from build123d import *

# Parameters (mm, degrees)
SALIENTE_EXTRUIR1_DEPTH      = 50
SALIENTE_EXTRUIR1_DEPTH_BACK = 7
CROQUIS1_W                   = 20
CROQUIS1_H                   = 20
CROQUIS2_R                   = 4
CORTAR_EXTRUIR1_DEPTH        = 58.445626465
CORTAR_EXTRUIR2_DEPTH        = 5
CROQUIS4_R                   = 4
CORTAR_EXTRUIR3_DEPTH        = 58.445626465
CORTAR_EXTRUIR4_DEPTH        = 5
REDONDEO1_R                  = 5
REDONDEO2_R                  = 1
REDONDEO3_R                  = 1


with BuildPart() as part:
    # Croquis1 → Saliente-Extruir1 (new, two sides: drawn at the far end of the back side and taken through both)
    with BuildSketch(Plane(origin=(0, 0, 0), x_dir=(1, 0, 0), z_dir=(0, 1, 0)).offset(-SALIENTE_EXTRUIR1_DEPTH_BACK)):
        with Locations((10, 10)):
            Rectangle(CROQUIS1_W, CROQUIS1_H)
    extrude(amount=SALIENTE_EXTRUIR1_DEPTH + SALIENTE_EXTRUIR1_DEPTH_BACK)

    # Croquis2 → Cortar-Extruir1 (cut, through all)
    with BuildSketch(Plane.XY):
        with Locations((10, 45)):
            Circle(CROQUIS2_R)
        with Locations((10, 20)):
            Circle(CROQUIS2_R)
    extrude(amount=-CORTAR_EXTRUIR1_DEPTH, mode=Mode.SUBTRACT)

    # Croquis3 → Cortar-Extruir2 (cut)
    with BuildSketch(Plane.XY):
        Polygon((13.92598183, 26.8), (6.07401817, 26.8), (2.148036339, 20), (6.07401817, 13.2), (13.92598183, 13.2), (17.851963661, 20), align=None)
    extrude(amount=-CORTAR_EXTRUIR2_DEPTH, mode=Mode.SUBTRACT)

    # Croquis4 → Cortar-Extruir3 (cut, through all)
    with BuildSketch(Plane.ZY):
        with Locations((-10, 30)):
            Circle(CROQUIS4_R)
        with Locations((-10, 10)):
            Circle(CROQUIS4_R)
    extrude(amount=-CORTAR_EXTRUIR3_DEPTH, mode=Mode.SUBTRACT)

    # Croquis5 → Cortar-Extruir4 (cut)
    with BuildSketch(Plane.ZY):
        Polygon((-6.07401817, 23.2), (-2.148036339, 30), (-6.07401817, 36.8), (-13.92598183, 36.8), (-17.851963661, 30), (-13.92598183, 23.2), align=None)
        Polygon((-6.07401817, 16.8), (-13.92598183, 16.8), (-17.851963661, 10), (-13.92598183, 3.2), (-6.07401817, 3.2), (-2.148036339, 10), align=None)
    extrude(amount=-CORTAR_EXTRUIR4_DEPTH, mode=Mode.SUBTRACT)

    # Redondeo1
    redondeo1_edges = [part.edges().sort_by_distance(p)[0] for p in [
        (0, 50, -10),
        (20, 50, -10),
    ]]
    fillet(redondeo1_edges, radius=REDONDEO1_R)

    # Redondeo2
    redondeo2_edges = [part.edges().sort_by_distance(p)[0] for p in [
        (20, -7, -10),
        (10, -7, -20),
        (0, -7, -10),
        (10, -7, 0),
    ]]
    fillet(redondeo2_edges, radius=REDONDEO2_R)

    # Redondeo3
    # the kernel refuses this fillet: 1 mm, written as the material it takes off along each edge
    with BuildSketch(Plane(origin=(19, -6, -19), x_dir=(0, 0, -1), z_dir=(1, 0, 0))) as redondeo3_piece_1_section:
        Polygon((0, 0), (REDONDEO3_R, 0), (REDONDEO3_R, -REDONDEO3_R), (0, -REDONDEO3_R), align=None)
    redondeo3_piece_1 = extrude(amount=REDONDEO3_R, mode=Mode.PRIVATE)
    redondeo3_piece_1 = redondeo3_piece_1 - Plane(origin=(19, -6, -19), x_dir=(0, 0.7071067811865475, 0.7071067811865475), z_dir=(1, 0, 0)) * Sphere(REDONDEO3_R, mode=Mode.PRIVATE)
    add(redondeo3_piece_1, mode=Mode.SUBTRACT)
    with BuildSketch(Plane(origin=(19, -6, -1), x_dir=(1, 0, 0), z_dir=(0, 0, 1))) as redondeo3_piece_2_section:
        Polygon((0, 0), (REDONDEO3_R, 0), (REDONDEO3_R, -REDONDEO3_R), (0, -REDONDEO3_R), align=None)
    redondeo3_piece_2 = extrude(amount=REDONDEO3_R, mode=Mode.PRIVATE)
    redondeo3_piece_2 = redondeo3_piece_2 - Plane(origin=(19, -6, -1), x_dir=(-0.7071067811865475, 0.7071067811865475, 0), z_dir=(0, 0, 1)) * Sphere(REDONDEO3_R, mode=Mode.PRIVATE)
    add(redondeo3_piece_2, mode=Mode.SUBTRACT)
    with BuildSketch(Plane(origin=(1, -6, -19), x_dir=(0, 0, -1), z_dir=(-1, 0, 0))) as redondeo3_piece_3_section:
        Polygon((0, 0), (REDONDEO3_R, 0), (REDONDEO3_R, REDONDEO3_R), (0, REDONDEO3_R), align=None)
    redondeo3_piece_3 = extrude(amount=REDONDEO3_R, mode=Mode.PRIVATE)
    redondeo3_piece_3 = redondeo3_piece_3 - Plane(origin=(1, -6, -19), x_dir=(0, 0.7071067811865475, 0.7071067811865475), z_dir=(-1, 0, 0)) * Sphere(REDONDEO3_R, mode=Mode.PRIVATE)
    add(redondeo3_piece_3, mode=Mode.SUBTRACT)
    with BuildSketch(Plane(origin=(1, -6, -1), x_dir=(-1, 0, 0), z_dir=(0, 0, 1))) as redondeo3_piece_4_section:
        Polygon((0, 0), (REDONDEO3_R, 0), (REDONDEO3_R, REDONDEO3_R), (0, REDONDEO3_R), align=None)
    redondeo3_piece_4 = extrude(amount=REDONDEO3_R, mode=Mode.PRIVATE)
    redondeo3_piece_4 = redondeo3_piece_4 - Plane(origin=(1, -6, -1), x_dir=(0.7071067811865475, 0.7071067811865475, 0), z_dir=(0, 0, 1)) * Sphere(REDONDEO3_R, mode=Mode.PRIVATE)
    add(redondeo3_piece_4, mode=Mode.SUBTRACT)
    with BuildSketch(Plane(origin=(5, 50, 0), x_dir=(0, -1, 0), z_dir=(1, 0, 0))) as redondeo3_piece_5:
        with BuildLine():
            CenterArc((REDONDEO3_R, REDONDEO3_R), REDONDEO3_R, 180, 90)
            Line((0, REDONDEO3_R), (0, 0))
            Line((0, 0), (REDONDEO3_R, 0))
        make_face()
    extrude(amount=10, mode=Mode.SUBTRACT)
    with BuildSketch(Plane(origin=(15, 50, -20), x_dir=(0, 0, 1), z_dir=(-1, 0, 0))) as redondeo3_piece_6:
        with BuildLine():
            CenterArc((REDONDEO3_R, -REDONDEO3_R), REDONDEO3_R, 90, 90)
            Line((0, -REDONDEO3_R), (0, 0))
            Line((0, 0), (REDONDEO3_R, 0))
        make_face()
    extrude(amount=10, mode=Mode.SUBTRACT)
    with BuildSketch(Plane(origin=(5, 45, -20), x_dir=(-1, 0, 0), z_dir=(0, -1, 0))) as redondeo3_piece_7:
        with BuildLine():
            CenterArc((5 - REDONDEO3_R, -REDONDEO3_R), REDONDEO3_R, 0, 90)
            Line((5 - REDONDEO3_R, 0), (5, 0))
            Line((5, 0), (5, -REDONDEO3_R))
        make_face()
    revolve(axis=Axis((5, 45, -20), (0, 0, -1)), revolution_arc=90, mode=Mode.SUBTRACT)
    with BuildSketch(Plane(origin=(15, 45, -20), x_dir=(0, 1, 0), z_dir=(-1, 0, 0))) as redondeo3_piece_8:
        with BuildLine():
            CenterArc((5 - REDONDEO3_R, -REDONDEO3_R), REDONDEO3_R, 0, 90)
            Line((5 - REDONDEO3_R, 0), (5, 0))
            Line((5, 0), (5, -REDONDEO3_R))
        make_face()
    revolve(axis=Axis((15, 45, -20), (0, 0, -1)), revolution_arc=90, mode=Mode.SUBTRACT)
    with BuildSketch(Plane(origin=(5, 45, 0), x_dir=(-1, 0, 0), z_dir=(0, -1, 0))) as redondeo3_piece_9:
        with BuildLine():
            CenterArc((5 - REDONDEO3_R, REDONDEO3_R), REDONDEO3_R, 270, 90)
            Line((5, REDONDEO3_R), (5, 0))
            Line((5, 0), (5 - REDONDEO3_R, 0))
        make_face()
    revolve(axis=Axis((5, 45, 0), (0, 0, -1)), revolution_arc=90, mode=Mode.SUBTRACT)
    with BuildSketch(Plane(origin=(15, 45, 0), x_dir=(0, 1, 0), z_dir=(-1, 0, 0))) as redondeo3_piece_10:
        with BuildLine():
            CenterArc((5 - REDONDEO3_R, REDONDEO3_R), REDONDEO3_R, 270, 90)
            Line((5, REDONDEO3_R), (5, 0))
            Line((5, 0), (5 - REDONDEO3_R, 0))
        make_face()
    revolve(axis=Axis((15, 45, 0), (0, 0, -1)), revolution_arc=90, mode=Mode.SUBTRACT)
    with BuildSketch(Plane(origin=(0, 45, 0), x_dir=(1, 0, 0), z_dir=(0, -1, 0)), Plane(origin=(0, 45, -20), x_dir=(0, 0, 1), z_dir=(0, -1, 0)), Plane(origin=(20, -6, -20), x_dir=(0, 0, 1), z_dir=(0, 1, 0)), Plane(origin=(20, -6, 0), x_dir=(-1, 0, 0), z_dir=(0, 1, 0))) as redondeo3_piece_11:
        with BuildLine():
            CenterArc((REDONDEO3_R, -REDONDEO3_R), REDONDEO3_R, 90, 90)
            Line((0, -REDONDEO3_R), (0, 0))
            Line((0, 0), (REDONDEO3_R, 0))
        make_face()
    extrude(amount=51, mode=Mode.SUBTRACT)


solid = part.part
Source: CAD feature listing. Evaluate the final solid. Frame: model axes, mm. A direction names the side the tool comes from. Round coordinates to 2 decimals unless told otherwise and drop trailing zeros. Loops run counter-clockwise (first coordinate to the right, second up) from the corner with the lowest first, then second, coordinate; pieces in that order, holes last. Notation, with made-up numbers: (23.5, 89.25) -> (75.5, 89.25) arc R3 cw to (75.5, 94.25) -> close; hole circle Ø10 at (-30.5, 70.25). An arc over 180 degrees is marked (long way). Answer as a JSON object with one key per item and string values. Group by question number.
Q1. Section query D-D (x = 17). State how many separate pieces and enclosed holes the cut face has, plus the area to 3 significant figures.
Q2. Contact query for flat-ended pins moving along their axis: P1, Ø1.5, axis at x = 2, z = -10.5, coming from the +Y side; P2, Ø4, axis at x = 7, y = 17, coming from the +Z side; P3, Ø10, axis at y = 11, z = -11, coming from the -X side. Output: stop coordinate, or through.
Q3. Section query B-B (z = -11.5). Output: boundary loops of the cut face in (x, y).
Q4. Section query A-A (x = 8.25). Output: boundary loops of the cut face in (y, z).
Q5. Ray query, line 1 (Y direction, x = 14.5, z = -9.25); line 2 (Y direction, x = 11, z = -12.75); line 3 (Y direction, x = 14.75, z = -12.5). Return the intervals inside material, ascending. Write a range as from..to.
Q6. Access query for faces 4 (the flat face through (15.92, 23.35, -2.46)), 5 (the cylindrical face through (0.285, 19.857, -19.699)), 6 (the flat face through (2.46, 33.35, -4.08)). Directions: +Z, -Z, +X, -X, +Y, -Y. A direction counts if a zero-diameter tool reaches every point of the face in a straight line with its end or side. Return the directions, or none.
Q7. Mould query, pull axis Z, two halves, no side actions, for faces 1 (the flat face through (2, 23.2, -10)), 2 (the flat face through (15.86, 16.55, -2.46)), 3 (the flat face through (5.9, 21.1, -20)). Classes: pulls with the +Z half, pulls with the -Z half, needs draft (parallel to the pull), parting line crosses it, or undercut.
Q8. Section query C-C (y = 8.5). Output: boundary loops of the cut face in (x, z), plus the area to 3 significant figures.
Completed:
{
 "1": {"separate pieces": "1", "enclosed holes": "2", "area": "1,020 mm²"},
 "2": {"P1": "y = 49.47", "P2": "z = -5", "P3": "x = 5"},
 "3": {"outline": "(0, -6) arc R1 ccw to (1, -7) -> (19, -7) arc R1 ccw to (20, -6) -> (20, 6.29) -> (5, 6.29) -> (5, 3.2) -> (0, 3.2) -> close; (0, 16.8) -> (5, 16.8) -> (5, 13.71) -> (20, 13.71) -> (20, 26.29) -> (5, 26.29) -> (5, 23.2) -> (0, 23.2) -> close; (0, 36.8) -> (5, 36.8) -> (5, 33.71) -> (20, 33.71) -> (20, 45) arc R5 ccw to (15, 50) -> (5, 50) arc R5 ccw to (0, 45) -> close; hole circle Ø8 at (10, 20); hole circle Ø8 at (10, 45)"},
 "4": {"outline": "(-7, -19) arc R1 ccw to (-6, -20) -> (16.4, -20) -> (16.4, -5) -> (13.2, -5) -> (13.2, 0) -> (-6, 0) arc R1 ccw to (-7, -1) -> close; (23.6, -20) -> (41.4, -20) -> (41.4, 0) -> (26.8, 0) -> (26.8, -5) -> (23.6, -5) -> close; (48.6, -20) -> (49, -20) arc R1 ccw to (50, -19) -> (50, -1) arc R1 ccw to (49, 0) -> (48.6, 0) -> close; hole circle Ø8 at (10, -10); hole circle Ø8 at (30, -10)"},
 "5": {"line 1": "-7..6.07, 13.93..26.07, 33.93..50", "line 2": "-7..7.1, 12.9..16.13, 23.87..27.1, 32.9..41.13, 48.87..50", "line 3": "-7..6.88, 13.12..26.88, 33.12..50"},
 "6": {"face 4": "+Z", "face 5": "-Z, -X, +Y, -Y", "face 6": "-X"},
 "7": {"face 1": "undercut", "face 2": "needs draft", "face 3": "pulls with the -Z half"},
 "8": {"outline": "(0, -19) arc R1 ccw to (1, -20) -> (19, -20) arc R1 ccw to (20, -19) -> (20, -13.71) -> (5, -13.71) -> (5, -16.99) -> (0, -16.99) -> close; (0, -3.01) -> (5, -3.01) -> (5, -6.29) -> (20, -6.29) -> (20, -1) arc R1 ccw to (19, 0) -> (1, 0) arc R1 ccw to (0, -1) -> close", "area": "218 mm²"}
}
